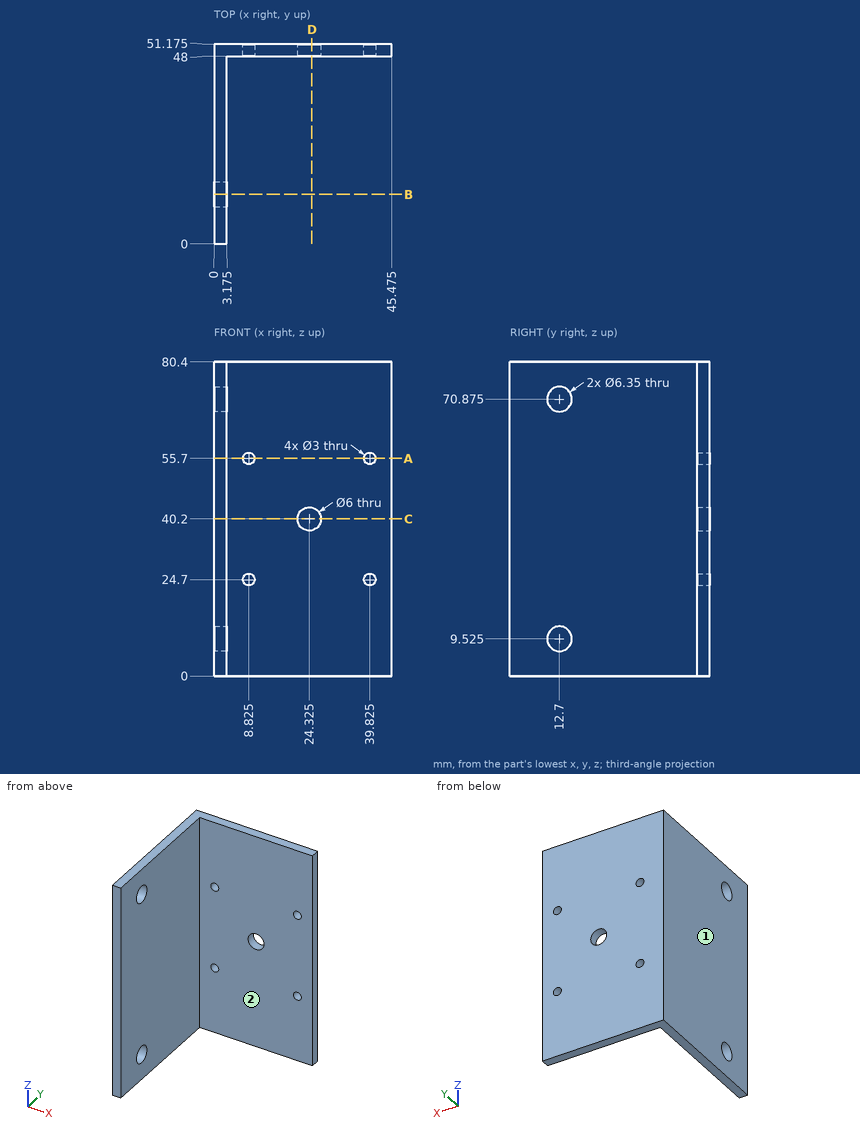
Geometry check sheet. Reference: drawing and pictorial views, mm from the part's lowest x, y, z. A direction names the side the tool comes from. Give positions to 0.01 mm unless a question says otherwise; leave off trailing zeros. Loops run counter-clockwise (first coordinate to the right, second up) from the corner with the lowest first, then second, coordinate; pieces in that order, holes last. Notation, with made-up numbers: M 4,-39.75 L 8,-39.75 A11 cw 8,-28.75 Z; hole C 79,51 d11. An arc over 180 degrees is marked long. One line per question, with ' | ' between items.
Item 1: Section check D-D, the plane x = 25. Record the cut outline in (y, z) (3 decimals).
Completed:
outline: M 48,0 L 51.175,0 L 51.175,37.277 L 48,37.277 Z; M 48,43.123 L 51.175,43.123 L 51.175,80.4 L 48,80.4 Z
Item 2: Tool access check on the marked faces 1 and 2. Record the directions out of +Z, -Z, +X, -X, +Y, -Y that give a thin tool (end or side, any length) a straight path to the whole face; none if there is none.
Completed:
face 1: +Z, -Z, -X, +Y, -Y | face 2: +Z, -Z, +X, -Y
Item 3: Depth check by flat-ended pin: P1, Ø2.5, axis at x = 8.825, z = 55.7, coming from the -Y side; P2, Ø6, axis at x = 23, z = 12, coming from the -Y side. Enter the tip coordinate at first touch or a pass-through.
Completed:
P1: passes through | P2: stops at y = 48
Item 4: Section check C-C, the plane z = 40.2. Record the cut outline in (x, y) (3 decimals), plus the area to 3 significant figures.
Completed:
outline: M 0,0 L 3.175,0 L 3.175,48 L 21.325,48 L 21.325,51.175 L 0,51.175 Z; M 27.325,48 L 45.475,48 L 45.475,51.175 L 27.325,51.175 Z | area: 278 mm^2
Item 5: Thickness scan on line 1 (X direction, y = 49.75, z = 24.7) (3 decimals); line 2 (X direction, y = 49, z = 55) (3 decimals); line 3 (Y direction, x = 10.5, z = 57.5) (3 decimals). Record the ranges inside material, lowest first. Write a range as [from, to].
Completed:
line 1: x = [0, 7.325], [10.325, 38.325], [41.325, 45.475] | line 2: x = [0, 7.498], [10.152, 38.498], [41.152, 45.475] | line 3: y = [48, 51.175]
Item 6: Section check B-B, the plane y = 12.7. Record the cut outline in (x, z) (3 decimals), plus the area to 3 significant figures.
Completed:
outline: M 0,0 L 3.175,0 L 3.175,6.35 L 0,6.35 Z; M 0,12.7 L 3.175,12.7 L 3.175,67.7 L 0,67.7 Z; M 0,74.05 L 3.175,74.05 L 3.175,80.4 L 0,80.4 Z | area: 215 mm^2
Item 7: Section check A-A, the plane z = 55.7. Record the cut outline in (x, y) (3 decimals).
Completed:
outline: M 0,0 L 3.175,0 L 3.175,48 L 7.325,48 L 7.325,51.175 L 0,51.175 Z; M 10.325,48 L 38.325,48 L 38.325,51.175 L 10.325,51.175 Z; M 41.325,48 L 45.475,48 L 45.475,51.175 L 41.325,51.175 Z
